from build123d import *

# Parameters (mm, degrees)
F0_R     = 6.35
F1_DEPTH = 1.5875
F2_W     = 482.6
F2_H     = 101.6
F2_R     = 6.35
F3_DEPTH = 1.5875


with BuildPart() as f1:
    # F0 (on Front) → F1 (new body)
    with BuildSketch(Plane.XZ):
        Polygon((0, 304.8), (0, 0), (482.6, 0), (482.6, 304.8), (349.25, 304.8), (336.55, 304.8), (146.05, 304.8), align=None)
        with Locations((19.05, 50.8)):
            Circle(F0_R, mode=Mode.SUBTRACT)
        with BuildLine():
            ThreePointArc((139.677532, 63.87253), (106.72929, 64.453708), (74.253289, 70.042424))
            ThreePointArc((74.253289, 70.042424), (69.647088, 77.751374), (77.356037, 82.357576))
            ThreePointArc((77.356037, 82.357576), (107.921685, 77.097608), (138.931795, 76.550617))
            ThreePointArc((138.931795, 76.550617), (145.643707, 70.584442), (139.677532, 63.87253))
        make_face(mode=Mode.SUBTRACT)
        with BuildLine():
            ThreePointArc((405.243963, 82.357576), (412.952912, 77.751374), (408.346711, 70.042424))
            ThreePointArc((408.346711, 70.042424), (375.87071, 64.453708), (342.922468, 63.87253))
            ThreePointArc((342.922468, 63.87253), (336.956293, 70.584442), (343.668205, 76.550617))
            ThreePointArc((343.668205, 76.550617), (374.678315, 77.097608), (405.243963, 82.357576))
        make_face(mode=Mode.SUBTRACT)
        with Locations((463.55, 50.8)):
            Circle(F0_R, mode=Mode.SUBTRACT)
        with Locations((19.05, 152.4)):
            Circle(F0_R, mode=Mode.SUBTRACT)
        with Locations((19.05, 254)):
            Circle(F0_R, mode=Mode.SUBTRACT)
        with Locations((127, 279.4)):
            Circle(F0_R, mode=Mode.SUBTRACT)
        with BuildLine():
            Line((146.05, 165.1), (146.05, 266.7))
            Line((146.05, 266.7), (336.55, 266.7))
            Line((336.55, 266.7), (336.55, 165.1))
            ThreePointArc((336.55, 165.1), (317.951281, 120.198719), (273.05, 101.6))
            Line((273.05, 101.6), (209.55, 101.6))
            ThreePointArc((209.55, 101.6), (164.648719, 120.198719), (146.05, 165.1))
        make_face(mode=Mode.SUBTRACT)
        with Locations((463.55, 152.4)):
            Circle(F0_R, mode=Mode.SUBTRACT)
        with Locations((355.6, 279.4)):
            Circle(F0_R, mode=Mode.SUBTRACT)
        with Locations((463.55, 254)):
            Circle(F0_R, mode=Mode.SUBTRACT)
    extrude(amount=F1_DEPTH)

    # F2 (on face) → F3 (join)
    with BuildSketch(Plane.XZ.offset(1.5875)):
        with Locations((241.3, 355.6)):
            Rectangle(F2_W, F2_H)
        with Locations((19.05, 355.6)):
            Circle(F2_R, mode=Mode.SUBTRACT)
        with Locations((463.55, 355.6)):
            Circle(F2_R, mode=Mode.SUBTRACT)
    extrude(amount=-F3_DEPTH)


solid = f1.part
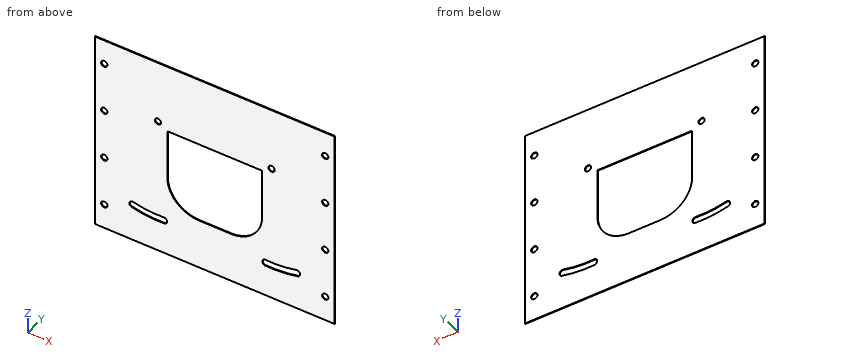
Could you check a few things on this model? Use its own coordinates, in mm. Coordinates: 2 decimals unless noted, no trailing zeros. Order: outer loops, then holes, each group sorted by start corner. A loop starts at its lowest first (then second) coordinate and runs counter-clockwise, first axis right, second up. Notation, with made-up numbers: (-5.5, 22) - (20.5, 22) arc R17 ccw to (20.5, 43) - close; hole circle Ø7 at (73, 76.25). An arc over 180 degrees is marked (long way). Answer in a Markdown table with one row per item. Add a question column.
(1) If we section it at A-A, the plane x = 463.55: Please give me the cut outline in (y, z).
(2) If we section it at D-D, the plane z = 194: Please give me the cut outline in (x, y).
(3) If we section it at C-C, the plane z = 279.4: Please give me the cut outline in (x, y).
(4) Will these pins go through, and if not, where does the flat tip stop? pin 1 (3 mm diameter, centred on x = 377, z = 350.5, fed in from +Y); pin 2 (11.5 mm diameter, centred on x = 127, z = 279.4, fed in from +Y).
(5) If we section it at B-B, the plane x = 355.6: Please give me the cut outline in (y, z), then the cut area to 3 significant figures.
(6) I need wall thicknesses on L1, parallel to Z at x = 463.55, y = -1.15; L2, parallel to Z at x = 355.6, y = -0.6; L3, parallel to X at y = -0.45, z = 181. Which ranges of each line are inside material? Lowest first, please.
Results are:
| question | item | result |
|---|---|---|
| 1 | outline | (-1.59, 0) - (0, 0) - (0, 44.45) - (-1.59, 44.45) - close; (-1.59, 57.15) - (0, 57.15) - (0, 146.05) - (-1.59, 146.05) - close; (-1.59, 158.75) - (0, 158.75) - (0, 247.65) - (-1.59, 247.65) - close; (-1.59, 260.35) - (0, 260.35) - (0, 349.25) - (-1.59, 349.25) - close; (-1.59, 361.95) - (0, 361.95) - (0, 406.4) - (-1.59, 406.4) - close |
| 2 | outline | (0, -1.59) - (146.05, -1.59) - (146.05, 0) - (0, 0) - close; (336.55, -1.59) - (482.6, -1.59) - (482.6, 0) - (336.55, 0) - close |
| 3 | outline | (0, -1.59) - (120.65, -1.59) - (120.65, 0) - (0, 0) - close; (133.35, -1.59) - (349.25, -1.59) - (349.25, 0) - (133.35, 0) - close; (361.95, -1.59) - (482.6, -1.59) - (482.6, 0) - (361.95, 0) - close |
| 4 | pin 1 | stops at y = 0 |
| 4 | pin 2 | passes through |
| 5 | outline | (-1.59, 0) - (0, 0) - (0, 63.5) - (-1.59, 63.5) - close; (-1.59, 76.2) - (0, 76.2) - (0, 273.05) - (-1.59, 273.05) - close; (-1.59, 285.75) - (0, 285.75) - (0, 406.4) - (-1.59, 406.4) - close |
| 5 | area | 605 mm2 |
| 6 | L1 | z = 0 to 44.45, 57.15 to 146.05, 158.75 to 247.65, 260.35 to 349.25, 361.95 to 406.4 |
| 6 | L2 | z = 0 to 63.5, 76.2 to 273.05, 285.75 to 406.4 |
| 6 | L3 | x = 0 to 146.05, 336.55 to 482.6 |
